The figure shows three views and two pictorial views of one solid part (mm, origin at its lowest corner). Answer the questions. A direction names the side the tool comes from. Give positions to 0.01 mm unless a question says otherwise; leave off trailing zeros. Loops run counter-clockwise (first coordinate to the right, second up) from the corner with the lowest first, then second, coordinate; pieces in that order, holes last. Notation, with made-up numbers: (-8, -15) - (34, -15) arc R18 cw to (34, -1) - close; hole circle Ø4 at (67, -20). An arc over 180 degrees is marked (long way). Write each question's results on one line, items separated by ' | '.
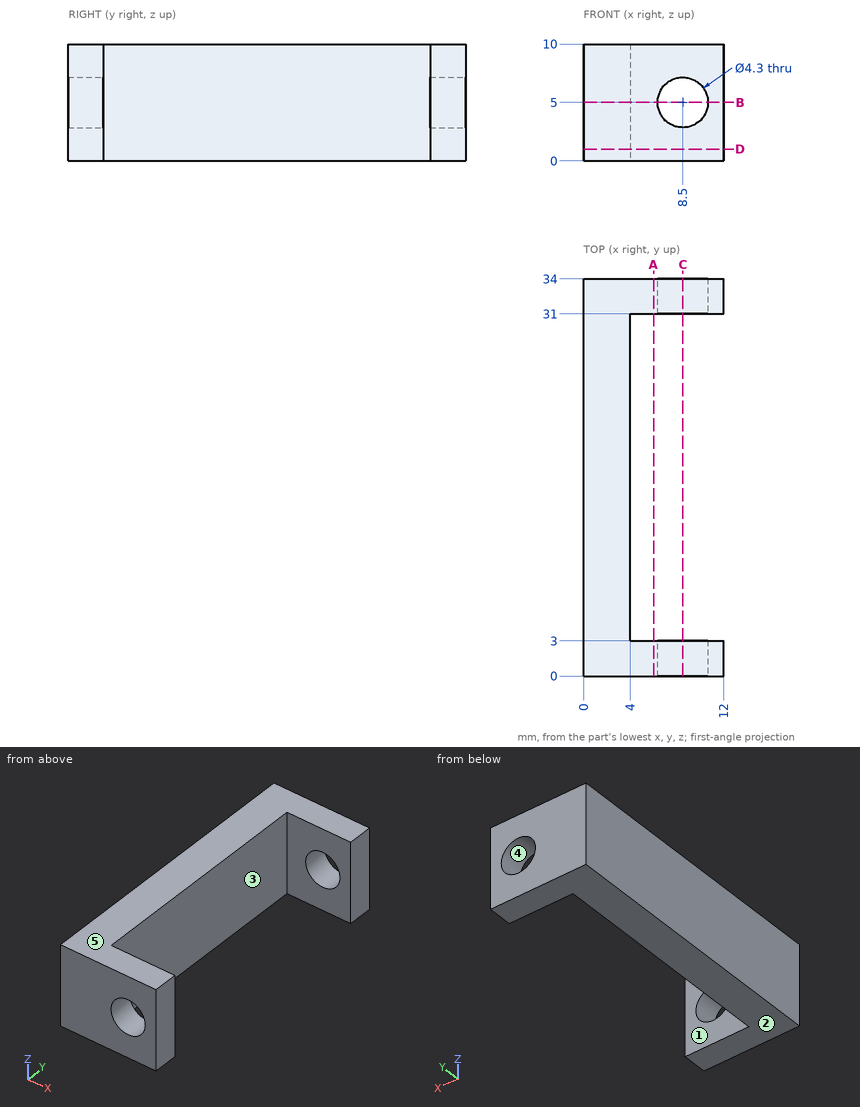
Item 1: A cutting plane is placed at A-A, the plane x = 6. Determine the outline of the cut face in (y, z), plus the area to 3 significant figures.
Values found:
outline: (0, 0) - (3, 0) - (3, 10) - (0, 10) - close; (31, 0) - (34, 0) - (34, 10) - (31, 10) - close | area: 60.0 mm²
Item 2: A flat-ended cylindrical pin translates along its axis: P1, Ø3, axis at y = 11.5, z = 2.5, coming from the +X side. Find the tip coordinate at first contact, or state that the pin passes through.
Values found:
P1: stops at x = 4
Item 3: A cutting plane is placed at D-D, the plane z = 1. Determine the outline of the cut face in (x, y), plus the area to 3 significant figures.
Values found:
outline: (0, 0) - (12, 0) - (12, 3) - (4, 3) - (4, 31) - (12, 31) - (12, 34) - (0, 34) - close | area: 184 mm²
Item 4: For the marked faces 1 and 2, determine the directions among +Z, -Z, +X, -X, +Y, -Y from which every point of the face is accessible in a straight line to the end or side of a thin tool.
Values found:
face 1: +Z, -Z, +X | face 2: -Z, +X, -X, +Y, -Y
Item 5: Find the intervals of material crossed by line 1 along Y through (x, z) = (10.75, 5.75); line 2 along Z through (x, y) = (8.5, 1); line 3 along X through (y, z) = (32.85, 5), in increasing order. Write a range as [from, to].
Values found:
line 1: y = [0, 3], [31, 34] | line 2: z = [0, 2.85], [7.15, 10] | line 3: x = [0, 6.35], [10.65, 12]
Item 6: A cutting plane is placed at B-B, the plane z = 5. Determine the outline of the cut face in (x, y), plus the area to 3 significant figures.
Values found:
outline: (0, 0) - (6.35, 0) - (6.35, 3) - (4, 3) - (4, 31) - (6.35, 31) - (6.35, 34) - (0, 34) - close; (10.65, 0) - (12, 0) - (12, 3) - (10.65, 3) - close; (10.65, 31) - (12, 31) - (12, 34) - (10.65, 34) - close | area: 158 mm²
Item 7: A cutting plane is placed at C-C, the plane x = 8.5. Determine the outline of the cut face in (y, z), plus the area to 3 significant figures.
Values found:
outline: (0, 0) - (3, 0) - (3, 2.85) - (0, 2.85) - close; (0, 7.15) - (3, 7.15) - (3, 10) - (0, 10) - close; (31, 0) - (34, 0) - (34, 2.85) - (31, 2.85) - close; (31, 7.15) - (34, 7.15) - (34, 10) - (31, 10) - close | area: 34.2 mm²
Item 8: For a pull along Z with two mould halves and no side action, classify the marked faces 3, 4 and 5 as released by +Z, released by -Z, zero draft, split by the parting line, or undercut.
Values found:
face 3: zero draft | face 4: undercut | face 5: released by +Z
